Geometry check sheet. Reference: the model listing, model coordinates, mm. A direction names the side the tool comes from. Give positions to 0.01 mm unless a question says otherwise; leave off trailing zeros. Write each loop counter-clockwise with the first axis right and the second up, starting at its lowest first coordinate (ties: lowest second). Pieces come first, ordered by that corner, then holes. Notation, with made-up numbers: (-39, -28) - (11, -28) arc R22 cw to (11, -19) - close; hole circle Ø10 at (47, 86.5). An arc over 180 degrees is marked (long way). Write item = value, one per line. Start each with the question number.
(1) Section check B-B, the plane z = 22. Enter the section's corners in (x, y).
(2) Depth check by flat-ended pin: pin 1 Ø2 at (x, y) = (4.5, 114.5) entering from -Z; pin 2 Ø6.5 at (x, y) = (6.5, 136.5) entering from -Z (3 decimals); pin 3 Ø4 at (x, y) = (3.5, 65) entering from +Z; pin 4 Ø6 at (x, z) = (10, 22.5) entering from +Y. Enter the tip coordinate at first touch or a pass-through.
(3) Section check C-C, the plane y = 131. Enter the section's corners in (x, z) (3 decimals), plus the area to 3 significant figures.
(4) Thickness scan on L1, parallel to Z at x = 6, y = 138.5 (3 decimals); L2, parallel to Z at x = 5, y = 54; L3, parallel to Y at x = 2.25, z = 24.5. Record the ranges inside material, lowest first.
(5) Section check A-A, the plane x = 11.25. Enter the section's corners in (y, z) (3 decimals).
(6) Access from +Z, -Z, +X, -X, +Y, -Y to the whole of each face (thin tool, end or side, straight path). Record for faces 1 (the flat face through (6, 140, 6.35)), 2 (the flat face through (6, 127, 2)), 3 (the flat face through (12.7, 58, 17)).
```python
from build123d import *

# Parameters (mm, degrees)
F1_DEPTH = 12.7
F2_R     = 25.4
F3_W     = 12.7
F3_H     = 3.175
F4_DEPTH = 25.4


with BuildPart() as f1:
    # F0 (on Right) → F1 (new body)
    with BuildSketch(Plane.YZ):
        Polygon((0, 6.35), (0, 0), (127, 0), (127, 6.35), (50.8, 50.344091), align=None)
    extrude(amount=F1_DEPTH)

    # F2
    f2_edges = [f1.edges().sort_by_distance(p)[0] for p in [
        (6.35, 50.8, 50.344091),
    ]]
    fillet(f2_edges, radius=F2_R)

    # F3 (on face) → F4 (join)
    with BuildSketch(Plane(origin=(0, 127, 0), x_dir=(-1, 0, 0), z_dir=(0, 1, 0))):
        with Locations((-6.35, 4.7625)):
            Rectangle(F3_W, F3_H)
    extrude(amount=F4_DEPTH)


solid = f1.part
```
Model answer:
q1.outline = (0, 18.07) - (12.7, 18.07) - (12.7, 99.89) - (0, 99.89) - close
q2.pin_1 = 0
q2.pin_2 = 3.175
q2.pin_3 = 42.97
q2.pin_4 = 104.22
q3.outline = (0, 3.175) - (12.7, 3.175) - (12.7, 6.35) - (0, 6.35) - close
q3.area = 40.3 mm²
q4.L1 = 3.175 to 6.35
q4.L2 = 0 to 44.7
q4.L3 = 20.96 to 95.56
q5.outline = (0, 0) - (127, 0) - (127, 3.175) - (152.4, 3.175) - (152.4, 6.35) - (127, 6.35) - (66.459, 41.303) arc R25.4 ccw to (37.131, 38.507) - (0, 6.35) - close
q6.face_1 = +Z, +X, -X, +Y
q6.face_2 = -Z, +X, -X, +Y
q6.face_3 = +Z, -Z, +X, +Y, -Y
